```python
from build123d import *
from OCP.BRepFilletAPI import BRepFilletAPI_MakeChamfer

# Parameters (mm, degrees)
SKETCH1_R               = 2.85
BOSS_EXTRUDE1_DEPTH     = 8
CUT_EXTRUDE1_REACH      = 22.027
CUT_EXTRUDE1_END_RADIUS = 2.85
SKETCH2_R               = 2.55
CIRPATTERN1_COUNT       = 3
CHAMFER1_SIZE           = 0.4
CHAMFER1_SIZE2          = 1.098990968
FILLET1_R               = 2
SKETCH3_R               = 10
BOSS_EXTRUDE2_DEPTH     = 3
SKETCH4_R               = 8
SKETCH4_R_2             = 7
CUT_EXTRUDE2_DEPTH      = 3
CHAMFER3_SIZE           = 3
CHAMFER2_SIZE           = 0.5


with BuildPart() as part:
    # Sketch1 → Boss-Extrude1 (new body)
    with BuildSketch(Plane(origin=(0, 0, 0), x_dir=(1, 0, 0), z_dir=(0, 1, 0))):
        Polygon((-4.58993464, 7.95), (4.58993464, 7.95), (9.17986928, 0), (4.58993464, -7.95), (-4.58993464, -7.95), (-9.17986928, 0), align=None)
        with Locations(Location((0, 0, 0), (0, 0, 270))):
            Circle(SKETCH1_R, mode=Mode.SUBTRACT)
    extrude(amount=BOSS_EXTRUDE1_DEPTH)

    # Cut-Extrude1: up to this cylinder (the profile starts outside it)
    cut_extrude1_end = Plane(origin=(0, 4, 0), z_dir=(0, -1, 0)) * Cylinder(CUT_EXTRUDE1_END_RADIUS, 50.754, mode=Mode.PRIVATE)
    # Sketch2 → Cut-Extrude1 (cut, up to the surface)
    with BuildSketch(Plane.XY.offset(7.95), mode=Mode.PRIVATE) as cut_extrude1_sk1:
        with Locations((0, 4)):
            Circle(SKETCH2_R)
    cut_extrude1_tool1 = extrude(cut_extrude1_sk1.sketch, amount=-CUT_EXTRUDE1_REACH, mode=Mode.PRIVATE) - cut_extrude1_end
    cut_extrude1 = cut_extrude1_tool1.solids().sort_by_distance((0, 4, 7.95))[0]
    add(cut_extrude1, mode=Mode.SUBTRACT)

    # CirPattern1: Cut-Extrude1 ×3 about axis
    cirpattern1_axis = Axis((0, 8, 0), (0, -1, 0))
    for i in range(1, CIRPATTERN1_COUNT):
        add(cut_extrude1.rotate(cirpattern1_axis, i * 360 / CIRPATTERN1_COUNT), mode=Mode.SUBTRACT)

    # Chamfer1: one chamfer whose edges measure the first distance from different faces: ONE call of the kernel's chamfer builder (chamfer() names one face for all edges)
    chamfer1_edges_1 = [part.edges().sort_by_distance(p)[0] for p in [
        (0, 8, -2.85),
    ]]
    chamfer1_side_1 = [part.faces().sort_by_distance(p)[0] for p in [
        (0, 8, -7.707123488),
    ]]
    chamfer1_edges_2 = [part.edges().sort_by_distance(p)[0] for p in [
        (-2.55, 4, 7.95),
    ]]
    chamfer1_side_2 = [part.faces().sort_by_distance(p)[0] for p in [
        (4.468168471, 4, 7.95),
    ]]
    chamfer1_edges_3 = [part.edges().sort_by_distance(p)[0] for p in [
        (-5.60990196, 4, -6.18336478),
    ]]
    chamfer1_side_3 = [part.faces().sort_by_distance(p)[0] for p in [
        (-9.118986195, 4, -0.105452596),
    ]]
    chamfer1_edges_4 = [part.edges().sort_by_distance(p)[0] for p in [
        (8.15990196, 4, -1.76663522),
    ]]
    chamfer1_side_4 = [part.faces().sort_by_distance(p)[0] for p in [
        (4.650817725, 4, -7.844547404),
    ]]
    chamfer1 = BRepFilletAPI_MakeChamfer(part.part.solid().wrapped)
    for e in chamfer1_edges_1:
        chamfer1.Add(CHAMFER1_SIZE, CHAMFER1_SIZE2, e.wrapped, chamfer1_side_1[0].wrapped)  # the first distance lies on this face
    for e in chamfer1_edges_2:
        chamfer1.Add(CHAMFER1_SIZE, CHAMFER1_SIZE2, e.wrapped, chamfer1_side_2[0].wrapped)  # the first distance lies on this face
    for e in chamfer1_edges_3:
        chamfer1.Add(CHAMFER1_SIZE, CHAMFER1_SIZE2, e.wrapped, chamfer1_side_3[0].wrapped)  # the first distance lies on this face
    for e in chamfer1_edges_4:
        chamfer1.Add(CHAMFER1_SIZE, CHAMFER1_SIZE2, e.wrapped, chamfer1_side_4[0].wrapped)  # the first distance lies on this face
    add(Compound.cast(chamfer1.Shape()), mode=Mode.REPLACE)

    # Fillet1
    fillet1_edges = [part.edges().sort_by_distance(p)[0] for p in [
        (-4.58993464, 4, 7.95),
        (-9.17986928, 4, 0),
        (-4.58993464, 4, -7.95),
        (4.58993464, 4, -7.95),
        (9.17986928, 4, 0),
        (4.58993464, 4, 7.95),
    ]]
    fillet(fillet1_edges, radius=FILLET1_R)

    # Sketch3 → Boss-Extrude2 (add)
    with BuildSketch(Plane.XZ):
        with Locations(Location((0, 0, 0), (0, 0, 270))):
            Circle(SKETCH3_R)
    extrude(amount=BOSS_EXTRUDE2_DEPTH)

    # Sketch4 → Cut-Extrude2 (cut)
    with BuildSketch(Plane.XZ.offset(3)):
        with Locations(Location((0, 0, 0), (0, 0, 270))):
            Circle(SKETCH4_R)
        with Locations(Location((0, 0, 0), (0, 0, 270))):
            Circle(SKETCH4_R_2, mode=Mode.SUBTRACT)
    extrude(amount=-CUT_EXTRUDE2_DEPTH, mode=Mode.SUBTRACT)

    # Chamfer3
    chamfer3_edges = [part.edges().sort_by_distance(p)[0] for p in [
        (0, -3, 7),
    ]]
    chamfer(chamfer3_edges, length=CHAMFER3_SIZE - 0.0001)  # a hair under: the kernel refuses the full size

    # Chamfer2
    chamfer2_edges = [part.edges().sort_by_distance(p)[0] for p in [
        (-6.88490196, 8, 3.975),
        (-6.88490196, 8, -3.975),
        (0, 8, 7.95),
        (6.88490196, 8, 3.975),
        (6.88490196, 8, -3.975),
        (0, 8, -7.95),
        (4.435234102, 8, -7.682050808),
        (-4.435234102, 8, -7.682050808),
        (8.870468203, 8, 0),
        (4.435234102, 8, 7.682050808),
        (-4.435234102, 8, 7.682050808),
        (-8.870468203, 8, 0),
    ]]
    chamfer(chamfer2_edges, length=CHAMFER2_SIZE)


solid = part.part
```
Could you check a few things on this model? Use its own coordinates, in mm. A direction names the side the tool comes from. Coordinates: 2 decimals unless noted, no trailing zeros. Write each loop counter-clockwise with the first axis right and the second up, starting at its lowest first coordinate (ties: lowest second). Pieces come first, ordered by that corner, then holes. Notation, with made-up numbers: (7, 0) -> (54, 0) arc R20 cw to (54, 7) -> close; hole circle Ø9 at (-40, 75). An arc over 180 degrees is marked (long way). Write item = value, one per line. Start each with the question number.
(1) Will these pins go through, and if not, where does the flat tip stop? pin 1 (3.5 mm diameter, centred on x = -1, y = 3, fed in from -Z); pin 2 (1.7 mm diameter, centred on x = 1, z = 0, fed in from +Y); pin 3 (6 mm diameter, centred on y = 4, z = 1.5, fed in from +X).
(2) I want a section at B-B (y = -0.75). Please give me the cut outline in (x, z), plus the area to 3 significant figures.
(3) I need wall thicknesses on line 1 (X direction, y = 1.2, z = 0); line 2 (Z direction, x = -5.75, y = -0.5); line 3 (Z direction, x = 0, y = 6.15). Which ranges of each line are inside material? Lowest first, please. Write a range as [from, to].
(4) I want a section at A-A (y = 0.75). Please give me the cut outline in (x, z).
(5) We'd pull the mould along X, two halves only. Please class faces 5 (the face through (2.43, 4.77, 4.78)), 6 (the face through (0.1, 8, -3.4)), 7 (the face through (-6.641, 7.754, 3.89)): released by +X, released by -X, zero draft, split by the parting line, or undercut.
(6) I want a section at C-C (x = 6.75). Give the number of separate pieces and of enclosed holes in the cut face, plus the area to 3 significant figures.
(7) Which directions (+Z, -Z, +X, -X, +Y, -Y) give clear straight access to the entire face, cutting with the end or side of a thin tool? Please do faces 1 (the face through (-8.87, 3.8, -0.01)), 2 (the face through (0, 4, -7.95)), 3 (the face through (2.403, 6.006, 1.532)), 4 (the face through (-5.315, 3.936, -6.694)).
Result set:
q1.pin_1 = -7.95
q1.pin_2 = 0
q1.pin_3 = 8.87
q2.outline = circle Ø20 at (0, 0); circle Ø12.5 at (0, 0); hole circle Ø16 at (0, 0)
q2.area = 236 mm2
q3.line_1 = [-8.87, -2.85], [2.85, 8.87]
q3.line_2 = [-8.18, -5.56], [-3.03, 3.03], [5.56, 8.18]
q3.line_3 = [-7.95, -2.85]
q4.outline = (-8.6, -1) -> (-5.17, -6.95) arc R2 ccw to (-3.44, -7.95) -> (3.44, -7.95) arc R2 ccw to (5.17, -6.95) -> (8.6, -1) arc R2 ccw to (8.6, 1) -> (5.17, 6.95) arc R2 ccw to (3.44, 7.95) -> (-3.44, 7.95) arc R2 ccw to (-5.17, 6.95) -> (-8.6, 1) arc R2 ccw to start; hole circle Ø5.7 at (0, 0)
q5.face_5 = undercut
q5.face_6 = zero draft
q5.face_7 = released by -X
q6.separate_pieces = 3
q6.enclosed_holes = 0
q6.area = 71.7 mm2
q7.face_1 = -X, +Y
q7.face_2 = -Z, +X, -X, +Y
q7.face_3 = +Y
q7.face_4 = -Z, -X, +Y
